```python
from build123d import *

# Parameters (mm, degrees)
F0_R          = 1.1
F1_DEPTH      = 34.6
F1_DEPTH_BACK = 34.6
F2_DEPTH      = 38
F2_DEPTH_BACK = 38
F4_DEPTH      = 1.2
F5_W          = 3.4
F5_H          = 12
F5_W_2        = 1.2
F5_H_2        = 66.4
F6_DEPTH      = 1.2
F7_DEPTH      = 5
F7_DEPTH_BACK = 5
F8_DEPTH      = 3.5
F9_R          = 1


# Not quite as in the source:
# - a pattern or mirror of a feature is missing from the dataset's text; its kind, count and spacing are read off the source's solid
# - a feature names something its author has since deleted; it is built from what else it names


with BuildPart() as f1:
    # F0 (on Front) → F1 (new body, two sides)
    with BuildSketch(Plane.XZ) as f1_sk:
        with BuildLine():
            ThreePointArc((-12.2672023306, 9.9350791425), (-14.5172023306, 12.1850791425), (-16.7672023306, 9.9350791425))
            Line((-16.7672023306, 9.9350791425), (-16.7672023306, 0))
            Line((-16.7672023306, 0), (10.9618057992, 0))
            ThreePointArc((10.9618057992, 0), (12.9295104862, 1.6360189486), (11.1762294546, 3.5))
            Line((11.1762294546, 3.5), (-12.2672023306, 3.5))
            Line((-12.2672023306, 3.5), (-12.2672023306, 9.9350791425))
        make_face()
        with Locations((-14.5172023306, 9.9350791425)):
            Circle(F0_R, mode=Mode.SUBTRACT)
    extrude(amount=F1_DEPTH)
    extrude(f1_sk.sketch, amount=-F1_DEPTH_BACK)

    # F0 (on Front) → F2 (join, two sides)
    with BuildSketch(Plane.XZ) as f2_sk:
        with Locations((-14.5172023306, 9.9350791425)):
            Circle(F0_R)
    extrude(amount=F2_DEPTH)
    extrude(f2_sk.sketch, amount=-F2_DEPTH_BACK)

    # F3 (on face) → F4 (cut)
    with BuildSketch(Plane.YZ.offset(-12.2672023306)):
        Polygon((-33.2, 4.5), (-33.2, 3.5), (33.2, 3.5), (33.2, 8.5350791425), (-33.2, 8.5350791425), align=None)
    extrude(amount=-F4_DEPTH, mode=Mode.SUBTRACT)

    # F5 (on face) → F6 (cut)
    with BuildSketch(Plane.XY.offset(3.5)):
        Polygon((11.1762294546, 34.6), (2.9438750446, 34.6), (4.3438750446, 33.2), (11.1762294546, 26.36764559), align=None)
        Polygon((4.3438750446, 33.2), (-12.2672023306, 33.2), (-12.2672023306, -33.2), (4.3438750446, -33.2), (11.1762294546, -26.36764559), (11.1762294546, 26.36764559), align=None)
        with Locations((1.2438750446, -20.35)):
            Rectangle(F5_W, F5_H, mode=Mode.SUBTRACT)
        with Locations((1.2438750446, 20.35)):
            Rectangle(F5_W, F5_H, mode=Mode.SUBTRACT)
        with Locations((-12.8672023306, 0)):
            Rectangle(F5_W_2, F5_H_2)
        Polygon((12.9438750446, 24.6), (11.1762294546, 26.36764559), (11.1762294546, -26.36764559), (12.9438750446, -24.6), align=None)
    extrude(amount=-F6_DEPTH, mode=Mode.SUBTRACT)

    # F5 (on face) → F7 (cut, two sides)
    with BuildSketch(Plane.XY.offset(3.5)) as f7_sk:
        Polygon((12.9438750446, 34.6), (11.1762294546, 34.6), (11.1762294546, 26.36764559), (12.9438750446, 24.6), align=None)
        Polygon((12.9438750446, -24.6), (11.1762294546, -26.36764559), (11.1762294546, -34.6), (12.9438750446, -34.6), align=None)
        Polygon((11.1762294546, -26.36764559), (4.3438750446, -33.2), (2.9438750446, -34.6), (11.1762294546, -34.6), align=None)
    f7 = extrude(amount=-F7_DEPTH, mode=Mode.SUBTRACT) + extrude(f7_sk.sketch, amount=F7_DEPTH_BACK, mode=Mode.SUBTRACT)

    # F7_copies: F7 across plane
    add(f7.mirror(Plane.ZX), mode=Mode.SUBTRACT)

    # F5 (on face) → F8 (join)
    with BuildSketch(Plane.XY.offset(3.5)):
        with Locations((1.2438750446, 20.35)):
            Rectangle(F5_W, F5_H)
        with Locations((1.2438750446, -20.35)):
            Rectangle(F5_W, F5_H)
    extrude(amount=F8_DEPTH)

    # F9
    f9_edges = [f1.edges().sort_by_distance(p)[0] for p in [
        (1.243875, -26.35, 7),
        (2.943875, -20.35, 7),
        (1.243875, -14.35, 7),
        (-0.456125, -20.35, 7),
        (-0.456125, 20.35, 7),
        (1.243875, 14.35, 7),
        (2.943875, 20.35, 7),
        (1.243875, 26.35, 7),
    ]]
    fillet(f9_edges, radius=F9_R)


solid = f1.part
```
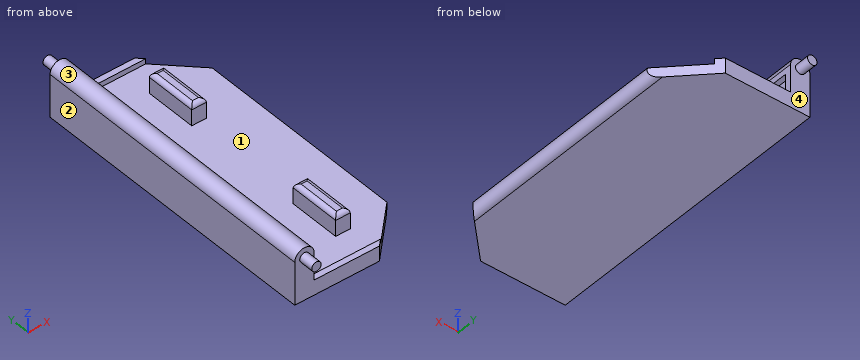
Could you check a few things on this model? Use its own coordinates, in mm. Face numbers are marked on the shaded views. Give positions to 0.01 mm unless a question says otherwise; leave off trailing zeros. Write each loop counter-clockwise with the first axis right and the second up, starting at its lowest first coordinate (ties: lowest second). Pieces come first, ordered by that corner, then holes. Notation, with made-up numbers: (85.5, -10.5) -> (122.5, -10.5) arc R8 cw to (122.5, -4.5) -> close; hole circle Ø6 at (36, 80). An arc over 180 degrees is marked (long way). Write each question's results on one line, items separated by ' | '.
1. Will these pins go through, and if not, where does the flat tip stop? pin 1 Ø10 at (x, y) = (-3, -9) entering from +Z; pin 2 Ø3 at (y, z) = (6.5, 8) entering from +X; pin 3 Ø2 at (y, z) = (27.5, 7) entering from +X.
Check sheet entries:
pin 1: stops at z = 2.3 | pin 2: stops at x = -12.27 | pin 3: stops at x = -13.47
2. I want a section at D-D, the plane z = 1.5. Write out the boundary of the cut face in (x, y), then the cut area to 3 significant figures.
Check sheet entries:
outline: (-16.77, -34.6) -> (2.94, -34.6) -> (12.92, -24.63) -> (12.92, 24.63) -> (2.94, 34.6) -> (-16.77, 34.6) -> close | area: 1,950 mm²
3. I want a section at B-B, the plane x = -8.5. Write out the boundary of the cut face in (y, z), then the cut area to 3 significant figures.
Check sheet entries:
outline: (-34.6, 0) -> (34.6, 0) -> (34.6, 3.5) -> (33.2, 3.5) -> (33.2, 2.3) -> (-33.2, 2.3) -> (-33.2, 3.5) -> (-34.6, 3.5) -> close | area: 163 mm²
4. I want a section at C-C, the plane y = -19.5. Write out the boundary of the cut face in (x, z), then the cut area to 3 significant figures.
Check sheet entries:
outline: (-16.77, 0) -> (10.96, 0) arc R1.76 ccw to (12.84, 2.3) -> (2.94, 2.3) -> (2.94, 6) arc R1 ccw to (1.94, 7) -> (0.54, 7) arc R1 ccw to (-0.46, 6) -> (-0.46, 2.3) -> (-13.47, 2.3) -> (-13.47, 8.54) -> (-12.27, 8.54) -> (-12.27, 9.94) arc R2.25 ccw to (-16.77, 9.94) -> close | area: 118 mm²
5. If we mould it in two halves opening along X, with no side actions, what happens to the marked faces 1, 2, 3 and 4? For each: released by +X, released by -X, zero draft, split by the parting line, or undercut.
Check sheet entries:
face 1: undercut | face 2: released by -X | face 3: split by the parting line | face 4: zero draft
6. I need wall thicknesses on L1, parallel to X at y = 16.5, z = 5.25; L2, parallel to Y at x = 0.75, z = 2.5; L3, parallel to X at y = 3, z = 3.5. Which ranges of each line are inside material? Lowest first, please.
Check sheet entries:
L1: x = -16.77 to -13.47, -0.46 to 2.94 | L2: y = -34.6 to -33.2, -26.35 to -14.35, 14.35 to 26.35, 33.2 to 34.6 | L3: x = -16.77 to -13.47
7. I want a section at A-A, the plane z = 5.25. Write out the boundary of the cut face in (x, y), then the cut area to 3 significant figures.
Check sheet entries:
outline: (-16.77, -34.6) -> (-12.27, -34.6) -> (-12.27, -33.2) -> (-13.47, -33.2) -> (-13.47, 33.2) -> (-12.27, 33.2) -> (-12.27, 34.6) -> (-16.77, 34.6) -> close; (-0.46, -26.35) -> (2.94, -26.35) -> (2.94, -14.35) -> (-0.46, -14.35) -> close; (-0.46, 14.35) -> (2.94, 14.35) -> (2.94, 26.35) -> (-0.46, 26.35) -> close | area: 313 mm²
